Design review of the part built by this model. Coordinates are the model's own, in mm. A direction names the side the tool comes from. Round coordinates to 2 decimals unless told otherwise and drop trailing zeros. Use CSV: the item, a comma, the result in double quotes. Start each with the question number.
from build123d import *


with BuildPart() as part:
    # Skizze1 → Rotation2 (revolve)
    with BuildSketch(Plane.XY, mode=Mode.PRIVATE) as rotation2_sk:
        Polygon((45.099637471, 45.974649946), (95.099637471, 45.974649946), (95.099637471, 70.974649946), (91.449637471, 70.974649946), (87.230554067, 57.174649946), (82.968720876, 57.174649946), (78.749637471, 70.974649946), (76.449637471, 70.974649946), (72.230554067, 57.174649946), (70.099637471, 57.174649946), (67.968720876, 57.174649946), (63.749637471, 70.974649946), (61.449637471, 70.974649946), (57.230554067, 57.174649946), (52.968720876, 57.174649946), (48.749637471, 70.974649946), (45.099637471, 70.974649946), align=None)
    revolve(rotation2_sk.sketch.rotate(Axis((24.821753872, 25.974649946, 0), (1, 0, 0)), 90), axis=Axis((24.821753872, 25.974649946, 0), (1, 0, 0)))  # turned: the seam where the file's is


solid = part.part
Q1. The part is to be moulded in two halves that separate along Y. For faces 1 (the cylindrical face through (70.45, 38.144, -15.871)), 2 (the conical face through (57.435, 16.402, 30.398)), 3 (the flat face through (95.1, 45, -9)), say which applies: +Y half, -Y half, draft (parallel to the pull), parting line (faces both ways), or undercut.
Q2. Take a section at B-B (y = -12.5). Give the number of separate pieces and of enclosed holes in the cut face, plus the area to 3 significant figures.
Q3. Clearance check with a flat-ended pin moving along its axis: pin 1 (4 mm diameter, centred on x = 90, y = 39, fed in from -Z). State where the tip first meets the part, or that it passes through.
Q4. Tool access review of faces 4 (the conical face through (82.705, 57.275, -6.951)), 5 (the cylindrical face through (46.9, 65.9, 20.76)): name each direction out of +Z, -Z, +X, -X, +Y, -Y from which nothing blocks a thin tool from reaching the whole face with its end or side.
Q5. For L1, parallel to Y at x = 55, z = 0; L2, parallel to X at y = -9.5, z = -19; L3, parallel to X at y = 56, z = 9.5, list the stretches that pass through material, from the lowest coordinate up. Write a range as [from, to].
Findings below:
1,face 1,"undercut"
1,face 2,"parting line"
1,face 3,"draft"
2,separate pieces,"4"
2,enclosed holes,"0"
2,area,"922 mm^2"
3,pin 1,"stops at z = -43.47"
4,face 4,"none"
4,face 5,"+X, -X"
5,L1,"y = [-5.23, 5.97], [45.97, 57.17]"
5,L2,"x = [45.1, 50.2], [60, 65.2], [75, 80.2], [90, 95.1]"
5,L3,"x = [45.1, 52.88], [57.32, 67.88], [72.32, 82.88], [87.32, 95.1]"
